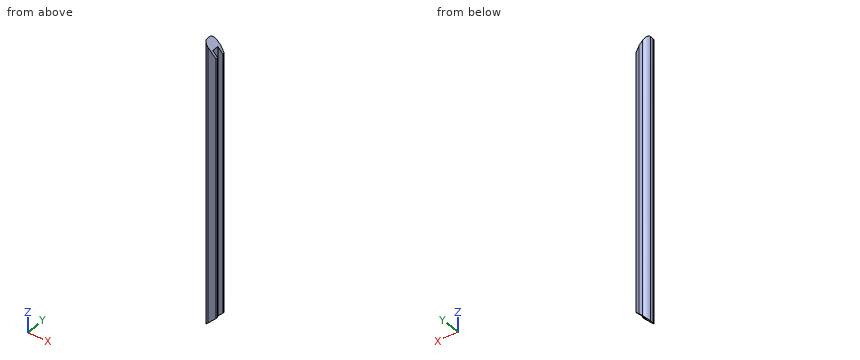
from build123d import *

# Parameters (mm, degrees)
SKETCH1_W           = 34.925
SKETCH1_H           = 34.925
BOSS_EXTRUDE1_DEPTH = 1320.8
SKETCH2_W           = 13.97
SKETCH2_H           = 19.05
CUT_EXTRUDE1_DEPTH  = 1322.030854224
FILLET1_R           = 12.7
CHAMFER1_SIZE       = 12.7
CHAMFER1_SIZE2      = 4.622421975
CUT_EXTRUDE2_DEPTH  = 1322.377059938


with BuildPart() as part:
    # Sketch1 → Boss-Extrude1 (new body)
    with BuildSketch(Plane.XY):
        Rectangle(SKETCH1_W, SKETCH1_H)
    extrude(amount=-BOSS_EXTRUDE1_DEPTH)

    # Sketch2 → Cut-Extrude1 (cut, through all)
    with BuildSketch(Plane.XY):
        with Locations((10.4775, -1.5875)):
            Rectangle(SKETCH2_W, SKETCH2_H)
    extrude(amount=-CUT_EXTRUDE1_DEPTH, mode=Mode.SUBTRACT)

    # Fillet1
    fillet1_edges = [part.edges().sort_by_distance(p)[0] for p in [
        (-17.4625, -17.4625, -660.4),
        (-17.4625, 17.4625, -660.4),
    ]]
    fillet(fillet1_edges, radius=FILLET1_R)

    # Chamfer1
    chamfer1_edges = [part.edges().sort_by_distance(p)[0] for p in [
        (17.4625, 17.4625, -660.4),
    ]]
    chamfer1_side = [part.faces().sort_by_distance(p)[0] for p in [
        (6.35, 17.4625, -660.4),
    ]]
    chamfer(chamfer1_edges, length=CHAMFER1_SIZE, length2=CHAMFER1_SIZE2, reference=chamfer1_side[0])

    # Sketch3 → Cut-Extrude2 (cut, through all)
    with BuildSketch(Plane(origin=(0, 17.4625, 0), x_dir=(1, 0, 0), z_dir=(0, 1, 0))):
        Polygon((-17.4625, 0), (17.4625, 34.925), (17.4625, 0), align=None)
        Polygon((-17.4625, 797.56), (17.4625, 762.635), (17.4625, 1320.8), (-17.4625, 1320.8), align=None)
    extrude(amount=-CUT_EXTRUDE2_DEPTH, mode=Mode.SUBTRACT)


solid = part.part
Part model, mm, in its own coordinate system. Give positions to 0.01 mm unless a question says otherwise; leave off trailing zeros. Loops run counter-clockwise (first coordinate to the right, second up) from the corner with the lowest first, then second, coordinate; pieces in that order, holes last.
(1) Pin check, flat tips, straight feed: pin 1 (5 mm diameter, centred on y = 11, z = -469.5, fed in from -X); pin 2 (5.5 mm diameter, centred on y = -4.5, z = -587, fed in from +X); pin 3 (7 mm diameter, centred on x = 9, z = -562.5, fed in from +Y). Stop position of each tip, or through.
Return value:
pin 1: stops at x = -16.9
pin 2: stops at x = 3.49
pin 3: stops at y = 17.19
(2) Band-saw the part on A-A (z = -49.5). Write the cut outline in (x, y), and give its area (3 significant figures).
Return value:
outline: (-17.46, -4.76) arc R12.7 ccw to (-4.76, -17.46) - (17.46, -17.46) - (17.46, -11.11) - (3.49, -11.11) - (3.49, 7.94) - (17.46, 7.94) - (17.46, 12.84) - (4.76, 17.46) - (-4.76, 17.46) arc R12.7 ccw to (-17.46, 4.76) - close
area: 855 mm2
(3) Band-saw the part on B-B (x = 11.5). Write the cut outline in (y, z), and give its area (3 significant figures).
Return value:
outline: (-17.46, -768.6) - (-11.11, -768.6) - (-11.11, -28.96) - (-17.46, -28.96) - close; (7.94, -768.6) - (15.01, -768.6) - (15.01, -28.96) - (7.94, -28.96) - close
area: 9,930 mm2
(4) Drill centre lines: line 1 along Y through (x, z) = (8, -174); line 2 along X through (y, z) = (0, -126.5); line 3 along Y through (x, z) = (-6, -161.5). Where is each one in solid material? Low to high.
Return value:
line 1: y = -17.46 to -11.11, 7.94 to 16.28
line 2: x = -17.46 to 3.49
line 3: y = -17.4 to 17.4
